Could you check a few things on this drawing? It's one solid part, dimensions in mm from its lowest x, y, z. Give positions to 0.01 mm unless a question says otherwise; leave off trailing zeros. Loops run counter-clockwise (first coordinate to the right, second up) from the corner with the lowest first, then second, coordinate; pieces in that order, holes last. Notation, with made-up numbers: M 71,69 L 76,69 A19 ccw 76,81 Z; hole C 61.5,79.5 d3. An arc over 180 degrees is marked long. Answer in a Markdown table with one row per item. Add a question column.
1. If we section it at C-C on y = 1.1: List the corners of the cut face in (x, z) for me (3 decimals).
2. If we section it at B-B on z = 33.3: List the corners of the cut face in (x, y) for me (3 decimals), then the cut area to 3 significant figures.
3. I need wall thicknesses on line 1 along Z through (x, y) = (12, 1.25) (3 decimals); line 2 along X through (y, z) = (0.55, 33); line 3 along Z through (x, y) = (47, 1.1). Which ranges of each line are inside material? Lowest first, please. Write a range as from..to.
4. If we section it at D-D on x = 47.5: List the corners of the cut face in (y, z) for me, then the cut area to 3 significant figures.
5. If we section it at A-A on x = 12: List the corners of the cut face in (y, z) for me (3 decimals), then the cut area to 3 significant figures.
6. I'm going to push a flat-ended pin straight in: pin 1 Ø2.5 at (x, z) = (39, 33.3) entering from +Y. Where does the tip first touch, or does it pass through?
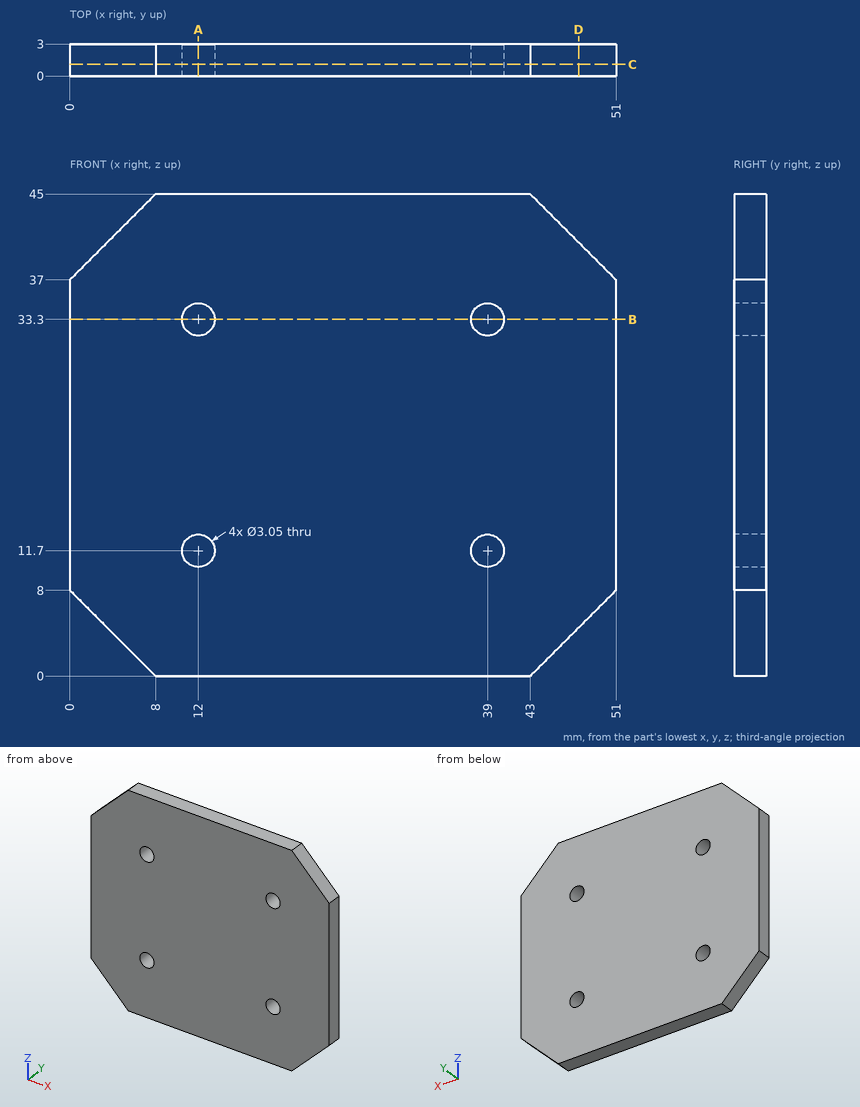
Results:
| question | item | result |
|---|---|---|
| 1 | outline | M 0,8 L 8,0 L 43,0 L 51,8 L 51,37 L 43,45 L 8,45 L 0,37 Z; hole C 12,11.7 d3.05; hole C 12,33.3 d3.05; hole C 39,11.7 d3.05; hole C 39,33.3 d3.05 |
| 2 | outline | M 0,0 L 10.475,0 L 10.475,3 L 0,3 Z; M 13.525,0 L 37.475,0 L 37.475,3 L 13.525,3 Z; M 40.525,0 L 51,0 L 51,3 L 40.525,3 Z |
| 2 | area | 135 mm2 |
| 3 | line 1 | 0..10.175, 13.225..31.775, 34.825..45 |
| 3 | line 2 | 0..10.5, 13.5..37.5, 40.5..51 |
| 3 | line 3 | 4..41 |
| 4 | outline | M 0,4.5 L 3,4.5 L 3,40.5 L 0,40.5 Z |
| 4 | area | 108 mm2 |
| 5 | outline | M 0,0 L 3,0 L 3,10.175 L 0,10.175 Z; M 0,13.225 L 3,13.225 L 3,31.775 L 0,31.775 Z; M 0,34.825 L 3,34.825 L 3,45 L 0,45 Z |
| 5 | area | 117 mm2 |
| 6 | pin 1 | through |
